from build123d import *

# Parameters (mm, degrees)
SKETCH_1_W               = 170
SKETCH_1_H               = 90
EXTRUDE_1_DEPTH          = 35
SKETCH_2_W               = 85
SKETCH_2_H               = 30
CUT_EXTRUDE_1_DEPTH      = 165
SKETCH_3_W               = 70.129701139
SKETCH_3_H               = 70.327043484
SKETCH_3_W_2             = 70.299701721
CUT_EXTRUDE_2_DEPTH      = 10
SKETCH_7_W               = 20
SKETCH_7_H               = 10
CUT_EXTRUDE_3_DEPTH      = 10
EXTRUDE_2_DEPTH          = 85
EXTRUDE_2_DEPTH_BACK     = 40
SKETCH_8_W               = 10
SKETCH_8_H               = 26.54076927
SKETCH_9_W               = 8.585786438
SKETCH_9_H               = 23.712342146
CUT_EXTRUDE_4_DEPTH      = 122
CUT_EXTRUDE_5_DEPTH      = 122
SKETCH_11_W              = 2
SKETCH_11_H              = 1.496455469
SKETCH_11_H_2            = 1.5
EXTRUDE_3_DEPTH          = 122
SKETCH_13_W              = 4
SKETCH_13_H              = 20
EXTRUDE_4_DEPTH          = 10
SKETCH_14_W              = 2
SKETCH_14_H              = 17.171572876
CUT_EXTRUDE_6_DEPTH      = 5
CUT_EXTRUDE_7_DEPTH      = 139.325702601
CUT_EXTRUDE_7_DEPTH_BACK = 5
SKETCH_16_R              = 2.5
SKETCH_16_R_2            = 5
EXTRUDE_5_DEPTH          = 32


with BuildPart() as part:
    # Эскиз1 → Бобышка-Вытянуть1 (new body)
    with BuildSketch(Plane(origin=(0, 0, 0), x_dir=(1, 0, 0), z_dir=(0, 1, 0))):
        Rectangle(SKETCH_1_W, SKETCH_1_H)
    extrude(amount=EXTRUDE_1_DEPTH)

    # Эскиз2 → Вырез-Вытянуть1 (cut)
    with BuildSketch(Plane(origin=(85, 0, 0), x_dir=(0, 0, -1), z_dir=(1, 0, 0))):
        with Locations((0, 17.5)):
            Rectangle(SKETCH_2_W, SKETCH_2_H)
    extrude(amount=-CUT_EXTRUDE_1_DEPTH, mode=Mode.SUBTRACT)

    # Эскиз3 → Вырез-Вытянуть2 (cut)
    with BuildSketch(Plane(origin=(0, 35, 0), x_dir=(1, 0, 0), z_dir=(0, 1, 0))):
        with Locations((45.364552291, -0.163521742)):
            Rectangle(SKETCH_3_W, SKETCH_3_H)
        with Locations((-39.850149139, -0.163521742)):
            Rectangle(SKETCH_3_W_2, SKETCH_3_H)
    extrude(amount=-CUT_EXTRUDE_2_DEPTH, mode=Mode.SUBTRACT)

    # Эскиз7 → Вырез-Вытянуть3 (cut)
    with BuildSketch(Plane.XY.offset(45)):
        with Locations((59.089377198, 17.5)):
            Rectangle(SKETCH_7_W, SKETCH_7_H)
        with Locations((-20.910622802, 17.5)):
            Rectangle(SKETCH_7_W, SKETCH_7_H)
    extrude(amount=-CUT_EXTRUDE_3_DEPTH, mode=Mode.SUBTRACT)

    # Эскиз8 → Бобышка-Вытянуть2 (add, two sides: drawn at the far end of the back side and taken through both)
    with BuildSketch(Plane(origin=(0, 0, 0), x_dir=(0, 0, -1), z_dir=(1, 0, 0)).offset(-EXTRUDE_2_DEPTH_BACK)):
        with Locations((-50, 13.270384635)):
            Rectangle(SKETCH_8_W, SKETCH_8_H)
    extrude(amount=EXTRUDE_2_DEPTH + EXTRUDE_2_DEPTH_BACK)

    # Эскиз9 → Вырез-Вытянуть4 (cut)
    with BuildSketch(Plane(origin=(85, 0, 0), x_dir=(0, 0, -1), z_dir=(1, 0, 0))):
        with Locations((-49.292893219, 13.270384635)):
            Rectangle(SKETCH_9_W, SKETCH_9_H)
    extrude(amount=-CUT_EXTRUDE_4_DEPTH, mode=Mode.SUBTRACT)

    # Эскиз10 → Вырез-Вытянуть5 (cut)
    with BuildSketch(Plane(origin=(85, 0, 0), x_dir=(0, 0, -1), z_dir=(1, 0, 0))):
        Polygon((-53.585786438, 2.914213562), (-57.191351612, 2.914213562), (-57.191351612, 23.710872093), (-53.585786438, 23.630100239), align=None)
    extrude(amount=-CUT_EXTRUDE_5_DEPTH, mode=Mode.SUBTRACT)

    # Эскиз11 → Бобышка-Вытянуть3 (add)
    with BuildSketch(Plane(origin=(85, 0, 0), x_dir=(0, 0, -1), z_dir=(1, 0, 0))):
        with Locations((-50.585786438, 24.378327973)):
            Rectangle(SKETCH_11_W, SKETCH_11_H)
        with Locations((-50.585786438, 2.164213562)):
            Rectangle(SKETCH_11_W, SKETCH_11_H_2)
    extrude(amount=-EXTRUDE_3_DEPTH)

    # Эскиз13 → Бобышка-Вытянуть4 (add)
    with BuildSketch(Plane(origin=(85, 0, 0), x_dir=(0, 0, -1), z_dir=(1, 0, 0))):
        with Locations((40.5, 17.5)):
            Rectangle(SKETCH_13_W, SKETCH_13_H)
        with Locations((-40.5, 17.5)):
            Rectangle(SKETCH_13_W, SKETCH_13_H)
    extrude(amount=-EXTRUDE_4_DEPTH)

    # Эскиз14 → Вырез-Вытянуть6 (cut)
    with BuildSketch(Plane(origin=(85, 0, 0), x_dir=(0, 0, -1), z_dir=(1, 0, 0))):
        with Locations((-40.914213562, 17.5)):
            Rectangle(SKETCH_14_W, SKETCH_14_H)
        with Locations((40.914213562, 17.5)):
            Rectangle(SKETCH_14_W, SKETCH_14_H)
    extrude(amount=-CUT_EXTRUDE_6_DEPTH, mode=Mode.SUBTRACT)

    # Эскиз15 → Вырез-Вытянуть7 (cut, two sides: drawn at the far end of the back side and taken through both)
    with BuildSketch(Plane(origin=(-37, 0, 0), x_dir=(0, 0, -1), z_dir=(1, 0, 0)).offset(-CUT_EXTRUDE_7_DEPTH_BACK)):
        Polygon((-55, 23.661781445), (-53.585786438, 23.630100239), (-53.585786438, 25.126555708), (-51.585786438, 25.126555708), (-51.585786438, 1.414213562), (-53.585786438, 1.414213562), (-53.585786438, 2.914213562), (-55, 2.914213562), (-57.035298645, 2.914213562), (-57.035298645, 23.645940842), align=None)
    extrude(amount=CUT_EXTRUDE_7_DEPTH + CUT_EXTRUDE_7_DEPTH_BACK, mode=Mode.SUBTRACT)

    # Эскиз16 → Бобышка-Вытянуть5 (add)
    with BuildSketch(Plane(origin=(0, 2.5, 0), x_dir=(1, 0, 0), z_dir=(0, 1, 0))):
        with Locations(Location((-41.821245604, 38.912307884, 0), (0, 0, 90))):
            Circle(SKETCH_16_R)
        with Locations(Location((-41.821245604, -38.979762053, 0), (0, 0, 90))):
            Circle(SKETCH_16_R)
        with Locations(Location((2.5, 0, 0), (0, 0, 90))):
            Circle(SKETCH_16_R_2)
        with Locations(Location((45.226425125, 38.912307884, 0), (0, 0, 90))):
            Circle(SKETCH_16_R)
        with Locations(Location((45.226425125, -39.333951436, 0), (0, 0, 90))):
            Circle(SKETCH_16_R)
        with Locations(Location((2.5, 30, 0), (0, 0, 90))):
            Circle(SKETCH_16_R_2)
        with Locations(Location((2.5, -30, 0), (0, 0, 90))):
            Circle(SKETCH_16_R_2)
    extrude(amount=EXTRUDE_5_DEPTH)


solid = part.part
Here's how the part is built. I have some questions about the finished solid (model axes, mm). A direction names the side the tool comes from. Coordinates: 2 decimals unless noted, no trailing zeros. Order: outer loops, then holes, each group sorted by start corner. A loop starts at its lowest first (then second) coordinate and runs counter-clockwise, first axis right, second up. Notation, with made-up numbers: M 42.5,22 L 95.5,22 A20 cw 95.5,43 Z; hole C 32,89.5 d11. An arc over 180 degrees is marked long. Answer as CSV lines item,"result".
Item 1: On a 3-axis mill with a long thin cutter (end or side, diameter ignored), from which of +Z, -Z, +X, -X, +Y, -Y can I reach the whole of each face in a straight line? I mean faces 4 (the face through (80, 27.5, 41)), 5 (the face through (2.28, 17.29, 34.995)), 6 (the face through (-1, 0, 6)). Say none if no direction works.
Results found:
face 4,"+X"
face 5,"none"
face 6,"+Z, -Z, +X, -X, -Y"
Item 2: Imagine slicing it at B-B on z = 7.5. Write out the boundary of the cut face in (x, y), plus the area to 3 significant figures.
Results found:
outline,"M -85,0 L 85,0 L 85,2.5 L -80,2.5 L -80,32.5 L -75,32.5 L -75,35 L -85,35 Z; M -4.7,32.5 L 10.3,32.5 L 10.3,35 L -4.7,35 Z; M 80.43,32.5 L 85,32.5 L 85,35 L 80.43,35 Z"
area,"649 mm2"
Item 3: We'd pull the mould along Y, two halves only. Please class faces 1 (the face through (-1, 35, -1)), 2 (the face through (85, 33, 2)), 3 (the face through (83, 17, 39.914)): +Y half, -Y half, draft (parallel to the pull), parting line (faces both ways), or undercut.
Results found:
face 1,"+Y half"
face 2,"draft"
face 3,"undercut"
Item 4: Imagine slicing it at D-D on x = 2.5. Give the number of separate pieces and of enclosed holes in the cut face, plus the area to 3 significant figures.
Results found:
separate pieces,"1"
enclosed holes,"4"
area,"1,540 mm2"
Item 5: For pin 1 (5.5 mm diameter, centred on x = 83.5, y = 17.5, fed in from +Z); pin 2 (12 mm diameter, centred on y = 14.5, z = -21, fed in from +X); pin 3 (5 mm diameter, centred on y = 15.5, z = 49, fed in from -X), each with a flat end and sliding along its axis, tell me the tip position at first contact or that it passes through.
Results found:
pin 1,"z = 45"
pin 2,"x = 6.5"
pin 3,"x = -40"
Item 6: If I drill on line 1 (Z direction, x = 57, y = 3); line 2 (Z direction, x = 6, y = 20.5); line 3 (Y direction, x = -58, z = 40), over which ranges is the centre line in solid material (lowest first)?
Results found:
line 1,"-45 to -42.5, 42.5 to 45"
line 2,"-45 to -42.5, -33.57 to -26.43, -3.57 to 3.57, 26.43 to 33.57, 42.5 to 45"
line 3,"0 to 2.5, 32.5 to 35"
Item 7: Imagine slicing it at A-A on z = 30. Write out the boundary of the cut face in (x, y), plus the area to 3 significant figures.
Results found:
outline,"M -85,0 L 85,0 L 85,2.5 L 7.5,2.5 L 7.5,32.5 L 10.3,32.5 L 10.3,35 L -4.7,35 L -4.7,32.5 L -2.5,32.5 L -2.5,2.5 L -80,2.5 L -80,32.5 L -75,32.5 L -75,35 L -85,35 Z; M 80.43,32.5 L 85,32.5 L 85,35 L 80.43,35 Z"
area,"949 mm2"
